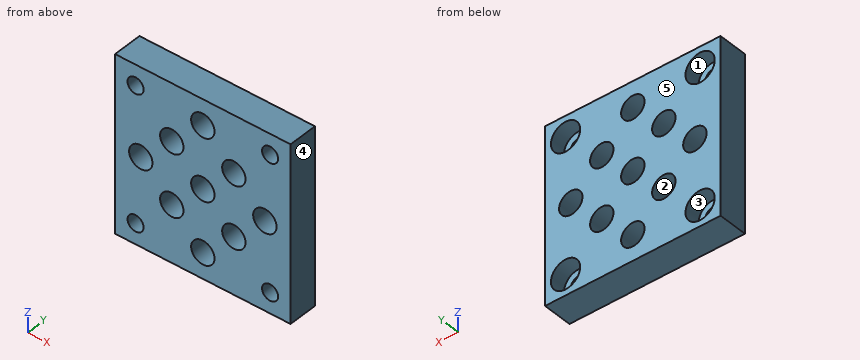
from build123d import *

# Parameters (mm, degrees)
CROQUIS1_W                                           = 60
CROQUIS1_H                                           = 60
SALIENTE_EXTRUIR1_DEPTH                              = 10
CROQUIS3_R                                           = 4
CORTAR_EXTRUIR2_DEPTH                                = 11
MATRIZL1_COUNT                                       = 3
MATRIZL1_PITCH                                       = 15
MATRIZL1_COUNT_DIR2                                  = 3
MATRIZL1_PITCH_DIR2                                  = 15
REFRENTADO_PARA_TORNILLO_CON_CABEZA_HUEC_D           = 5.5
REFRENTADO_PARA_TORNILLO_CON_CABEZA_HUEC_CBORE_D     = 10
REFRENTADO_PARA_TORNILLO_CON_CABEZA_HUEC_CBORE_DEPTH = 5.4


with BuildPart() as part:
    # Croquis1 → Saliente-Extruir1 (new body)
    with BuildSketch(Plane(origin=(0, 0, 0), x_dir=(1, 0, 0), z_dir=(0, 1, 0))):
        Rectangle(CROQUIS1_W, CROQUIS1_H)
    extrude(amount=SALIENTE_EXTRUIR1_DEPTH)

    # Croquis3 → Cortar-Extruir2 (cut, through all)
    with BuildSketch(Plane(origin=(0, 10, 0), x_dir=(1, 0, 0), z_dir=(0, 1, 0))):
        with Locations((0, -21.213203436)):
            Circle(CROQUIS3_R)
    cortar_extruir2 = extrude(amount=-CORTAR_EXTRUIR2_DEPTH, mode=Mode.SUBTRACT)

    # MatrizL1: Cortar-Extruir2 3 × 3
    with Locations(*[Vector(0.707106781, 0, -0.707106781) * (i * MATRIZL1_PITCH) + Vector(-0.707106781, 0, -0.707106781) * (j * MATRIZL1_PITCH_DIR2) for i in range(MATRIZL1_COUNT) for j in range(MATRIZL1_COUNT_DIR2) if (i, j) != (0, 0)]):
        add(cortar_extruir2, mode=Mode.SUBTRACT)

    # Refrentado para tornillo con cabeza hueca de M51 (through all)
    with Locations(Plane(origin=(-23, 10, -23), x_dir=(0, 0, 1), z_dir=(0, 1, 0))):
        with Locations((0, 0), (0, 46), (46, 46), (46, 0)):
            CounterBoreHole(REFRENTADO_PARA_TORNILLO_CON_CABEZA_HUEC_D / 2, REFRENTADO_PARA_TORNILLO_CON_CABEZA_HUEC_CBORE_D / 2, REFRENTADO_PARA_TORNILLO_CON_CABEZA_HUEC_CBORE_DEPTH)


solid = part.part
CAD build for the part. Positions are in the model's coordinates, mm. Face numbers are marked on the shaded views. A direction names the side the tool comes from. Round coordinates to 2 decimals unless told otherwise and drop trailing zeros. Order: outer loops, then holes, each group sorted by start corner. A loop starts at its lowest first (then second) coordinate and runs counter-clockwise, first axis right, second up. Notation, with made-up numbers: (18.25, -29) -> (77.25, -29) arc R23 cw to (77.25, -7) -> close; hole circle Ø2 at (-18, 41.5). An arc over 180 degrees is marked (long way). Write item = value, one per line. Start each with the question number.
(1) Which spindle directions (+Z, -Z, +X, -X, +Y, -Y) get a long thin tool onto all of the face, cutting with end or side? Do the marked faces 1 and 2. Say none if no direction does.
(2) Cut at A-A, the plane x = 0. List the corners of the cut face in (y, z), then the cut area to 3 significant figures.
(3) Pin check, flat tip, straight feed: P1, Ø9, axis at x = -23, z = -23, coming from the +Y side. Stop position of the tip, or through.
(4) Cut at D-D, the plane x = -9. List the corners of the cut face in (y, z).
(5) Cut at C-C, the plane z = 8.5. List the corners of the cut face in (x, y).
(6) Probe line 1 (X direction, y = 4, z = 12); line 2 (X direction, y = 4, z = -1); line 3 (X direction, y = 4.5, z = 0.5). List the from-to ranges inside material, lowest first. Write a range as [from, to].
(7) Pull direction X, two halves, no side cores. Call the marked faces 3, 4 and 5: released by +X, released by -X, zero draft, split by the parting line, or undercut.
(8) Cut at B-B, the plane z = 0. List the corners of the cut face in (x, y), then the cut area to 3 significant figures.
Model answer:
q1.face_1 = +Y
q1.face_2 = +Y, -Y
q2.outline = (0, -30) -> (10, -30) -> (10, -25.21) -> (0, -25.21) -> close; (0, -17.21) -> (10, -17.21) -> (10, -4) -> (0, -4) -> close; (0, 4) -> (10, 4) -> (10, 17.21) -> (0, 17.21) -> close; (0, 25.21) -> (10, 25.21) -> (10, 30) -> (0, 30) -> close
q2.area = 360 mm2
q3.P1 = 4.6
q4.outline = (0, -30) -> (10, -30) -> (10, -14.27) -> (0, -14.27) -> close; (0, -6.94) -> (10, -6.94) -> (10, 6.94) -> (0, 6.94) -> close; (0, 14.27) -> (10, 14.27) -> (10, 30) -> (0, 30) -> close
q5.outline = (-30, 0) -> (-14.01, 0) -> (-14.01, 10) -> (-30, 10) -> close; (-7.21, 0) -> (7.21, 0) -> (7.21, 10) -> (-7.21, 10) -> close; (14.01, 0) -> (30, 0) -> (30, 10) -> (14.01, 10) -> close
q6.line_1 = [-30, -14.36], [-6.86, 6.86], [14.36, 30]
q6.line_2 = [-30, -25.09], [-17.34, -3.87], [3.87, 17.34], [25.09, 30]
q6.line_3 = [-30, -25.18], [-17.24, -3.97], [3.97, 17.24], [25.18, 30]
q7.face_3 = undercut
q7.face_4 = released by +X
q7.face_5 = zero draft
q8.outline = (-30, 0) -> (-25.21, 0) -> (-25.21, 10) -> (-30, 10) -> close; (-17.21, 0) -> (-4, 0) -> (-4, 10) -> (-17.21, 10) -> close; (4, 0) -> (17.21, 0) -> (17.21, 10) -> (4, 10) -> close; (25.21, 0) -> (30, 0) -> (30, 10) -> (25.21, 10) -> close
q8.area = 360 mm2
